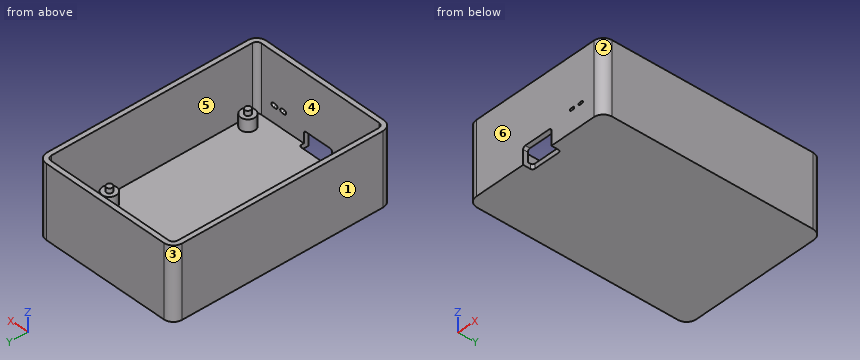
```python
from build123d import *

# Parameters (mm, degrees)
F0_W          = 62
F0_H          = 92
F1_DEPTH      = 2
F2_W          = 62
F2_H          = 92
F2_W_2        = 58
F2_H_2        = 88
F2_R          = 3
F3_DEPTH      = 28
F4_DEPTH      = 23
F5_R          = 1.25
F6_DEPTH      = 2
F7_R          = 1.25
F8_DEPTH      = 2
F9_R          = 1.25
F10_DEPTH     = 2
F11_R         = 1.25
F12_DEPTH     = 2
F14_DEPTH     = 4
F15_R         = 1
F16_R         = 2
F17_R         = 4
F18_T1_DEPTH  = 1
F18_T3_DEPTH  = 1
F18_T6_ANGLE  = 180
F18_T8_ANGLE  = 180
F18_T10_ANGLE = 180
F18_T12_ANGLE = 180


# Not quite as in the source:
# - a fillet or chamfer that OpenCascade refuses, or shapes differently, is made with other operations: its cross-section is extruded or revolved along the edge and cut away or added


with BuildPart() as f1:
    # F0 (on Top) → F1 (new body)
    with BuildSketch(Plane.XY):
        with Locations((31, 46)):
            Rectangle(F0_W, F0_H)
    extrude(amount=F1_DEPTH)

    # F2 (on face) → F3 (join)
    with BuildSketch(Plane.XY.offset(2)):
        with Locations((31, 46)):
            Rectangle(F2_W, F2_H)
        with Locations((31, 46)):
            Rectangle(F2_W_2, F2_H_2, mode=Mode.SUBTRACT)
        with Locations((7.5, 67)):
            Circle(F2_R)
        with Locations((56.5, 67)):
            Circle(F2_R)
        with Locations((7.5, 9)):
            Circle(F2_R)
        with Locations((56.5, 9)):
            Circle(F2_R)
    extrude(amount=F3_DEPTH)

    # F4 (cut): faces of the model
    f4_faces = [f1.faces().sort_by_distance(p)[0] for p in [
        (7.5, 67, 30),
        (56.5, 67, 30),
        (56.5, 9, 30),
        (7.5, 9, 30),
    ]]
    extrude(f4_faces, amount=-F4_DEPTH, mode=Mode.SUBTRACT)

    # F5 (on face) → F6 (join)
    with BuildSketch(Plane.XY.offset(7)):
        with Locations((7.5, 9)):
            Circle(F5_R)
    extrude(amount=F6_DEPTH)

    # F7 (on face) → F8 (join)
    with BuildSketch(Plane.XY.offset(7)):
        with Locations((56.5, 9)):
            Circle(F7_R)
    extrude(amount=F8_DEPTH)

    # F9 (on face) → F10 (join)
    with BuildSketch(Plane.XY.offset(7)):
        with Locations((56.5, 67)):
            Circle(F9_R)
    extrude(amount=F10_DEPTH)

    # F11 (on face) → F12 (join)
    with BuildSketch(Plane.XY.offset(7)):
        with Locations((7.5, 67)):
            Circle(F11_R)
    extrude(amount=F12_DEPTH)

    # F13 (on face) → F14 (cut)
    with BuildSketch(Plane.XZ):
        with BuildLine():
            ThreePointArc((38.5, 6), (38.2071067812, 6.7071067812), (37.5, 7))
            Line((37.5, 7), (26.5, 7))
            ThreePointArc((26.5, 7), (25.7928932188, 6.7071067812), (25.5, 6))
            Line((25.5, 6), (25.5, 0))
            Line((25.5, 0), (38.5, 0))
            Line((38.5, 0), (38.5, 6))
        make_face()
        with BuildLine():
            Line((48.5, 9.5), (47.5, 9.5))
            ThreePointArc((47.5, 9.5), (47.1464466094, 9.3535533906), (47, 9))
            ThreePointArc((47, 9), (47.1464466094, 8.6464466094), (47.5, 8.5))
            Line((47.5, 8.5), (48.5, 8.5))
            ThreePointArc((48.5, 8.5), (48.8535533906, 8.6464466094), (49, 9))
            ThreePointArc((49, 9), (48.8535533906, 9.3535533906), (48.5, 9.5))
        make_face()
        with BuildLine():
            Line((52.5, 9.5), (51.5, 9.5))
            ThreePointArc((51.5, 9.5), (51.1464466094, 9.3535533906), (51, 9))
            ThreePointArc((51, 9), (51.1464466094, 8.6464466094), (51.5, 8.5))
            Line((51.5, 8.5), (52.5, 8.5))
            ThreePointArc((52.5, 8.5), (52.8535533906, 8.6464466094), (53, 9))
            ThreePointArc((53, 9), (52.8535533906, 9.3535533906), (52.5, 9.5))
        make_face()
    extrude(amount=-F14_DEPTH, mode=Mode.SUBTRACT)

    # F15
    f15_edges = [f1.edges().sort_by_distance(p)[0] for p in [
        (25.5, 4, 1),
        (38.5, 4, 1),
    ]]
    fillet(f15_edges, radius=F15_R)

    # F16
    f16_edges = [f1.edges().sort_by_distance(p)[0] for p in [
        (2, 90, 16),
        (60, 90, 16),
        (60, 2, 16),
        (2, 2, 16),
    ]]
    fillet(f16_edges, radius=F16_R)

    # F17
    f17_edges = [f1.edges().sort_by_distance(p)[0] for p in [
        (0, 92, 15),
        (62, 92, 15),
        (62, 0, 15),
        (0, 0, 15),
    ]]
    fillet(f17_edges, radius=F17_R)

    # F18: chamfer of 1 x 0.3639702343 on 8 edges, made by hand

    # F18_s2 → F18_t1 (cut)
    with BuildSketch(Plane.YZ.offset(51.5)):
        Polygon((2, 9.8639702343), (1, 9.5), (2, 9.5), align=None)
        Polygon((2, 8.1360297657), (1, 8.5), (2, 8.5), align=None)
    extrude(amount=F18_T1_DEPTH, mode=Mode.SUBTRACT)

    # F18_s4 → F18_t3 (cut)
    with BuildSketch(Plane.YZ.offset(47.5)):
        Polygon((2, 9.8639702343), (1, 9.5), (2, 9.5), align=None)
        Polygon((2, 8.1360297657), (1, 8.5), (2, 8.5), align=None)
    extrude(amount=F18_T3_DEPTH, mode=Mode.SUBTRACT)

    # F18_s5 → F18_t6 (revolve, cut)
    with BuildSketch(Plane.YZ.offset(51.5)):
        Polygon((2, 9.8639702343), (1, 9.5), (2, 9.5), align=None)
    revolve(axis=Axis((51.5, 2, 9), (0, -1, 0)), revolution_arc=F18_T6_ANGLE, mode=Mode.SUBTRACT)

    # F18_s7 → F18_t8 (revolve, cut)
    with BuildSketch(Plane.YZ.offset(47.5)):
        Polygon((2, 9.8639702343), (1, 9.5), (2, 9.5), align=None)
    revolve(axis=Axis((47.5, 2, 9), (0, -1, 0)), revolution_arc=F18_T8_ANGLE, mode=Mode.SUBTRACT)

    # F18_s9 → F18_t10 (revolve, cut)
    with BuildSketch(Plane.YZ.offset(52.5)):
        Polygon((2, 8.1360297657), (1, 8.5), (2, 8.5), align=None)
    revolve(axis=Axis((52.5, 2, 9), (0, -1, 0)), revolution_arc=F18_T10_ANGLE, mode=Mode.SUBTRACT)

    # F18_s11 → F18_t12 (revolve, cut)
    with BuildSketch(Plane.YZ.offset(48.5)):
        Polygon((2, 8.1360297657), (1, 8.5), (2, 8.5), align=None)
    revolve(axis=Axis((48.5, 2, 9), (0, -1, 0)), revolution_arc=F18_T12_ANGLE, mode=Mode.SUBTRACT)


solid = f1.part
```
Geometry check sheet. Reference: the model listing, model coordinates, mm. Face numbers are marked on the shaded views. A direction names the side the tool comes from. Coordinates: 2 decimals unless noted, no trailing zeros. Loops run counter-clockwise (first coordinate to the right, second up) from the corner with the lowest first, then second, coordinate; pieces in that order, holes last. Notation, with made-up numbers: (51.5, 30) -> (84.5, 30) arc R23 ccw to (84.5, 57) -> close; hole circle Ø1 at (16, 18.5). An arc over 180 degrees is marked (long way). Put each result on its own line as item: value.
1) Thickness scan on line 1 (X direction, y = 59.5, z = 28.75); line 2 (Y direction, x = 20, z = 20); line 3 (Y direction, x = 8.5, z = 4.25). Record the ranges inside material, lowest first.
Result set:
line 1: x = 0 to 2, 60 to 62
line 2: y = 0 to 2, 90 to 92
line 3: y = 0 to 2, 6.17 to 11.83, 64.17 to 69.83, 90 to 92
2) Release check for a two-part mould opening along Y. For the marked faces 1, 2, 3 and 4 record: released by +Y, released by -Y, zero draft, split by the parting line, or undercut.
Result set:
face 1: zero draft
face 2: released by -Y
face 3: released by +Y
face 4: undercut
3) Cross-section at B-B on x = 23. Record the boundary of the cut face in (y, z), plus the area to 3 significant figures.
Result set:
outline: (0, 0) -> (92, 0) -> (92, 30) -> (90, 30) -> (90, 2) -> (2, 2) -> (2, 30) -> (0, 30) -> close
area: 296 mm^2
4) Tool access check on the marked faces 5 and 6. Record the directions out of +Z, -Z, +X, -X, +Y, -Y that give a thin tool (end or side, any length) a straight path to the whole face; none if there is none.
Result set:
face 5: +Z
face 6: +Z, -Z, +X, -X, -Y
5) Gauge pin test, flat ends, axial feed: pin 1 Ø3.5 at (y, z) = (1.5, 4) entering from +X; pin 2 Ø2 at (x, y) = (56.5, 67) entering from +Z; pin 3 Ø5 at (x, y) = (45, 9.5) entering from +Z. Record the tip position at first contact, or that the pin passes through.
Result set:
pin 1: stops at x = 61.93
pin 2: stops at z = 9
pin 3: stops at z = 2
6) Cross-section at C-C on y = 9. Record the boundary of the cut face in (x, z).
Result set:
outline: (0, 0) -> (62, 0) -> (62, 30) -> (60, 30) -> (60, 2) -> (59.5, 2) -> (59.5, 7) -> (57.75, 7) -> (57.75, 9) -> (55.25, 9) -> (55.25, 7) -> (53.5, 7) -> (53.5, 2) -> (10.5, 2) -> (10.5, 7) -> (8.75, 7) -> (8.75, 9) -> (6.25, 9) -> (6.25, 7) -> (4.5, 7) -> (4.5, 2) -> (2, 2) -> (2, 30) -> (0, 30) -> close
7) Cross-section at A-A on z = 21.5. Record the boundary of the cut face in (x, y), plus the area to 3 significant figures.
Result set:
outline: (0, 4) arc R4 ccw to (4, 0) -> (58, 0) arc R4 ccw to (62, 4) -> (62, 88) arc R4 ccw to (58, 92) -> (4, 92) arc R4 ccw to (0, 88) -> close; hole (2, 4) arc R2 ccw to (4, 2) -> (58, 2) arc R2 ccw to (60, 4) -> (60, 88) arc R2 ccw to (58, 90) -> (4, 90) arc R2 ccw to (2, 88) -> close
area: 590 mm^2
8) Cross-section at D-D on x = 7.5. Record the boundary of the cut face in (y, z).
Result set:
outline: (0, 0) -> (92, 0) -> (92, 30) -> (90, 30) -> (90, 2) -> (70, 2) -> (70, 7) -> (68.25, 7) -> (68.25, 9) -> (65.75, 9) -> (65.75, 7) -> (64, 7) -> (64, 2) -> (12, 2) -> (12, 7) -> (10.25, 7) -> (10.25, 9) -> (7.75, 9) -> (7.75, 7) -> (6, 7) -> (6, 2) -> (2, 2) -> (2, 30) -> (0, 30) -> close
